from build123d import *

# Parameters (mm, degrees)
SKETCH1_W           = 76
SKETCH1_H           = 76
SKETCH1_W_2         = 70
SKETCH1_H_2         = 70
BOSS_EXTRUDE1_DEPTH = 40
SKETCH2_W           = 70
SKETCH2_H           = 70
BOSS_EXTRUDE2_DEPTH = 3


with BuildPart() as part:
    # Sketch1 → Boss-Extrude1 (new body)
    with BuildSketch(Plane(origin=(0, 0, 0), x_dir=(1, 0, 0), z_dir=(0, 1, 0))):
        with Locations((35, 35)):
            Rectangle(SKETCH1_W, SKETCH1_H)
        with Locations((35, 35)):
            Rectangle(SKETCH1_W_2, SKETCH1_H_2, mode=Mode.SUBTRACT)
    extrude(amount=BOSS_EXTRUDE1_DEPTH)

    # Sketch2 → Boss-Extrude2 (add)
    with BuildSketch(Plane.XZ):
        with Locations((35, -35)):
            Rectangle(SKETCH2_W, SKETCH2_H)
    extrude(amount=-BOSS_EXTRUDE2_DEPTH)


solid = part.part
Work out the finished part from the listing and answer in its coordinate system (mm). A direction names the side the tool comes from. Round coordinates to 2 decimals unless told otherwise and drop trailing zeros. Loops run counter-clockwise (first coordinate to the right, second up) from the corner with the lowest first, then second, coordinate; pieces in that order, holes last. Notation, with made-up numbers: (9.5, -26.75) - (37.5, -26.75) arc R21 ccw to (37.5, -18.75) - close; hole circle Ø9 at (49, -32.75). An arc over 180 degrees is marked (long way). One line per item, written item: value.
Q1. Each of these flat-tipped pins is pushed along its axis until it touches: pin 1 Ø1 at (x, z) = (53, -61.5) entering from -Y; pin 2 Ø8 at (x, z) = (58, -32) entering from +Y. Where does it stop, or does it pass through?
Check values:
pin 1: y = 0
pin 2: y = 3
Q2. Straight lines are drawn through the part: probe 1 along X at (y, z) = (30.5, -61.5); probe 2 along Z at (x, y) = (8, 36); probe 3 along Y at (x, z) = (20, -68). For each, find the intervals that lie inside material, in ascending order.
Check values:
probe 1: -3 to 0, 70 to 73
probe 2: -73 to -70, 0 to 3
probe 3: 0 to 3
Q3. Find section A-A on y = 23.5. Give the vertices of the cut face in (x, z).
Check values:
outline: (-3, -73) - (73, -73) - (73, 3) - (-3, 3) - close; hole (0, -70) - (70, -70) - (70, 0) - (0, 0) - close
Q4. For faces 5 (the flat face through (35, 21, 0)), 6 (the flat face through (34, 20, -73)), determine the directions among +Z, -Z, +X, -X, +Y, -Y from which every point of the face is accessible in a straight line to the end or side of a thin tool.
Check values:
face 5: +Y
face 6: -Z, +X, -X, +Y, -Y
Q5. Find section B-B on x = 12. Give the vertices of the cut face in (y, z), and give its area (3 significant figures).
Check values:
outline: (0, -73) - (40, -73) - (40, -70) - (3, -70) - (3, 0) - (40, 0) - (40, 3) - (0, 3) - close
area: 450 mm2
Q6. Find section C-C on z = -35. Give the vertices of the cut face in (x, y), and give its area (3 significant figures).
Check values:
outline: (-3, 0) - (73, 0) - (73, 40) - (70, 40) - (70, 3) - (0, 3) - (0, 40) - (-3, 40) - close
area: 450 mm2
Q7. The mould has two halves that part along X. Classify faces 1 (the flat face through (-3, 20, -34)), 2 (the flat face through (34, 20, 3)), 3 (the flat face through (0, 21, -35)), 4 (the flat face through (73, 20, -34)): +X half, -X half, draft (parallel to the pull), parting line (faces both ways), or undercut.
Check values:
face 1: -X half
face 2: draft
face 3: undercut
face 4: +X half
